Part model, mm, in its own coordinate system. Give positions to 0.01 mm unless a question says otherwise; leave off trailing zeros. Order: outer loops, then holes, each group sorted by start corner. A loop starts at its lowest first (then second) coordinate and runs counter-clockwise, first axis right, second up. Notation, with made-up numbers: (21.5, -21) -> (78.5, -21) arc R16 ccw to (78.5, -8) -> close; hole circle Ø5 at (6, -11.75). An arc over 180 degrees is marked (long way). Write item = value, one per line. Start each with the question number.
(1) Flat gauge pins, fed straight in: pin 1 (8 mm diameter, centred on x = -25, z = 5.5, fed in from +Y); pin 2 (1 mm diameter, centred on y = 33.5, z = -1, fed in from -X); pin 3 (5 mm diameter, centred on x = -71.5, y = 72, fed in from +Z). Where does each tip first touch, or does it go through?
(2) Probe line 1 along Z through (x, y) = (58.5, 42) (1 decimal); line 2 along X through (y, z) = (19, 3.25); line 3 along X through (y, z) = (67, 7). List the from-to ranges inside material, lowest first. Write a range as from..to.
(3) Saw through at B-B, the plane z = -2. List the corners of the cut face in (x, y), then the cut area to 3 significant figures.
(4) Saw through at A-A, the plane x = 0. List the corners of the cut face in (y, z) (1 decimal), then the cut area to 3 significant figures.
from build123d import *

# Parameters (mm, degrees)
BOSS_EXTRUDE1_DEPTH = 5.715
BOSS_EXTRUDE2_DEPTH = 6.0325
BOSS_EXTRUDE3_START = 7.3025
BOSS_EXTRUDE3_DEPTH = 7.3025
FILLET1_R           = 2.54
SKETCH6_W           = 6.645493415
SKETCH6_H           = 6.096
CUT_EXTRUDE5_DEPTH  = 3.81


with BuildPart() as part:
    # Sketch1 → Boss-Extrude1 (new body)
    with BuildSketch(Plane.XY):
        with BuildLine():
            ThreePointArc((69.342, 73.406), (0, 4.064), (-69.342, 73.406))
            Line((-69.342, 73.406), (-73.406, 73.406))
            ThreePointArc((-73.406, 73.406), (0, 0), (73.406, 73.406))
            Line((73.406, 73.406), (69.342, 73.406))
        make_face()
    extrude(amount=BOSS_EXTRUDE1_DEPTH)

    # Sketch3 → Boss-Extrude2 (add)
    with BuildSketch(Plane.XY.offset(5.715)):
        with BuildLine():
            ThreePointArc((65.5955, 73.406), (0, 7.8105), (-65.5955, 73.406))
            Line((-65.5955, 73.406), (-69.342, 73.406))
            ThreePointArc((-69.342, 73.406), (0, 4.064), (69.342, 73.406))
            Line((69.342, 73.406), (65.5955, 73.406))
        make_face()
        with BuildLine():
            Line((73.406, 73.406), (69.342, 73.406))
            ThreePointArc((69.342, 73.406), (0, 4.064), (-69.342, 73.406))
            Line((-69.342, 73.406), (-73.406, 73.406))
            ThreePointArc((-73.406, 73.406), (0, 0), (73.406, 73.406))
        make_face()
    extrude(amount=BOSS_EXTRUDE2_DEPTH)

    # Sketch4 → Boss-Extrude3 (add)
    with BuildSketch(Plane(origin=(0, 0, 0), x_dir=(-1, 0, 0), z_dir=(0, 0, -1)).offset(BOSS_EXTRUDE3_START)):
        with BuildLine():
            ThreePointArc((65.5955, 73.406), (0, 7.8105), (-65.5955, 73.406))
            Line((-65.5955, 73.406), (-69.342, 73.406))
            ThreePointArc((-69.342, 73.406), (0, 4.064), (69.342, 73.406))
            Line((69.342, 73.406), (65.5955, 73.406))
        make_face()
        with BuildLine():
            Line((73.406, 73.406), (69.342, 73.406))
            ThreePointArc((69.342, 73.406), (0, 4.064), (-69.342, 73.406))
            Line((-69.342, 73.406), (-73.406, 73.406))
            ThreePointArc((-73.406, 73.406), (0, 0), (73.406, 73.406))
        make_face()
    extrude(amount=-BOSS_EXTRUDE3_DEPTH)

    # Fillet1
    fillet1_edges = [part.edges().sort_by_distance(p)[0] for p in [
        (0, 4.064, 5.715),
        (0, 4.064, 0),
    ]]
    fillet(fillet1_edges, radius=FILLET1_R)

    # Sketch6 → Cut-Extrude5 (cut)
    with BuildSketch(Plane.XY.offset(11.7475)):
        with Locations((-70.506627119, 70.358)):
            Rectangle(SKETCH6_W, SKETCH6_H)
        with Locations((70.506627119, 70.358)):
            Rectangle(SKETCH6_W, SKETCH6_H)
    extrude(amount=-CUT_EXTRUDE5_DEPTH, mode=Mode.SUBTRACT)


solid = part.part
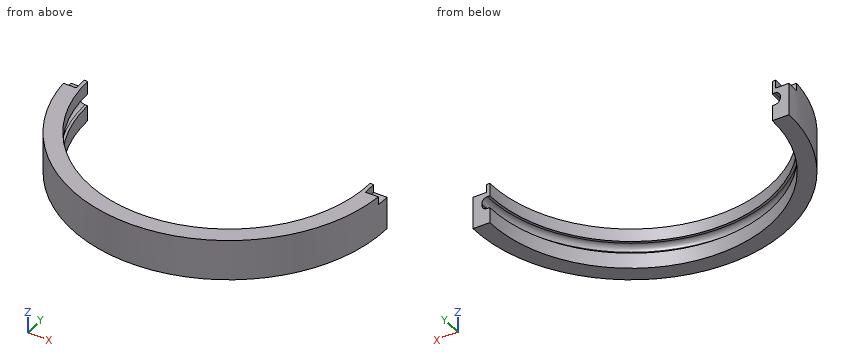
Results list:
q1.pin_1 = 14.57
q1.pin_2 = -61.93
q1.pin_3 = 7.94
q2.line_1 = -7.3..0, 5.7..11.7
q2.line_2 = -49.28..-42.99, 42.99..49.28
q2.line_3 = -73.13..-65.28, 65.28..73.13
q3.outline = (-73.41, 73.41) arc R73.41 ccw to (73.41, 73.41) -> (65.6, 73.41) arc R65.6 cw to (-65.6, 73.41) -> close
q3.area = 1,710 mm^2
q4.outline = (0, -7.3) -> (7.8, -7.3) -> (7.8, 0) -> (6.6, 0) arc R2.5 cw to (4.1, 2.5) -> (4.1, 3.2) arc R2.5 cw to (6.6, 5.7) -> (7.8, 5.7) -> (7.8, 11.7) -> (0, 11.7) -> close
q4.area = 130 mm^2
